Source: CAD feature listing. Evaluate the final solid. Frame: model axes, mm. A direction names the side the tool comes from. Round coordinates to 2 decimals unless told otherwise and drop trailing zeros. Order: outer loops, then holes, each group sorted by start corner. A loop starts at its lowest first (then second) coordinate and runs counter-clockwise, first axis right, second up. Notation, with made-up numbers: (-30, -17) - (-23, -17) arc R23 ccw to (-23, 0) - close; hole circle Ø2 at (84, 2). An arc over 180 degrees is marked (long way). Return JSON: item names as keys, results as strings. Group by question number.
1) Ray query, line 1 (Y direction, x = 32, z = 5); line 2 (X direction, y = 11, z = 5); line 3 (Y direction, x = 32, z = 8). Return the intervals inside material, ascending. Write a range as from..to.
2) Section C-C, the plane y = 10. Return loops of the section in (x, z), plus the area to 3 significant figures.
3) Section A-A, the plane z = 5.5. Give the number of separate pieces and of enclosed holes in the cut face, plus the area to 3 significant figures.
4) Section B-B, the plane y = 4. Return loops of the section in (x, z).
5) Access query for faces 4 (the flat face through (-4, 13, 3)), 5 (the flat face through (34, 13, 3)), 6 (the cylindrical face through (32, -2, 3)), 7 (the flat face through (30, 12, 3)). Directions: +Z, -Z, +X, -X, +Y, -Y. A direction counts if a zero-diameter tool reaches every point of the face in a straight line with its end or side. Return the directions, or none.
6) Section D-D, the plane x = -2. Return loops of the section in (y, z).
7) Contact query for flat-ended pins moving along their axis: P1, Ø3.5, axis at y = 12.5, z = 5, coming from the +X side; P2, Ø3, axis at x = 8, y = 23.5, coming from the -Z side; P3, Ø1, axis at x = 7.5, z = 5.5, coming from the +Y side. Output: stop coordinate, or through.
8) Mould query, pull axis Y, two halves, no side actions, for faces 1 (the cylindrical face through (-4.65, -4.49, 9.03)), 2 (the cylindrical face through (-0.5, 0.07, 5.42)), 3 (the flat face through (15, 32.5, 9)). Classes: pulls with the +Y half, pulls with the -Y half, needs draft (parallel to the pull), parting line crosses it, or undercut.
```python
from build123d import *

# Parameters (mm, degrees)
BOSS_EXTRUDE1_DEPTH   = 7
BOSS_EXTRUDE1_2_DEPTH = 7
SKETCH2_W             = 45
SKETCH2_H             = 40
BOSS_EXTRUDE2_DEPTH   = 4
FILLET1_R             = 10
SKETCH3_R             = 1.5
CUT_EXTRUDE1_DEPTH    = 16


with BuildPart() as part:
    # Sketch1 → Boss-Extrude1 (new body)
    with BuildSketch(Plane.XY):
        with BuildLine():
            Line((0, 0), (0, 25))
            ThreePointArc((0, 25), (-2, 27), (-4, 25))
            Line((-4, 25), (-4, 0))
            ThreePointArc((-4, 0), (-2, -2), (0, 0))
        make_face()
    extrude(amount=BOSS_EXTRUDE1_DEPTH)



with BuildPart() as body_2:
    # Sketch1 → Boss-Extrude1 2 (new body)
    with BuildSketch(Plane.XY):
        with BuildLine():
            Line((30, 0), (30, 25))
            ThreePointArc((30, 25), (32, 27), (34, 25))
            Line((34, 25), (34, 0))
            ThreePointArc((34, 0), (32, -2), (30, 0))
        make_face()
    extrude(amount=BOSS_EXTRUDE1_2_DEPTH)


with BuildPart() as part_1:
    add(part.part)

    add(body_2.part)  # Boss-Extrude2 merges body 2
    # Sketch2 → Boss-Extrude2 (add)
    with BuildSketch(Plane.XY.offset(7)):
        with Locations((15, 12.5)):
            Rectangle(SKETCH2_W, SKETCH2_H)
    extrude(amount=BOSS_EXTRUDE2_DEPTH)

    # Fillet1
    fillet1_edges = [part_1.edges().sort_by_distance(p)[0] for p in [
        (37.5, -7.5, 9),
        (37.5, 32.5, 9),
        (-7.5, 32.5, 9),
        (-7.5, -7.5, 9),
    ]]
    fillet(fillet1_edges, radius=FILLET1_R)

    # Sketch3 → Cut-Extrude1 (cut)
    with BuildSketch(Plane(origin=(0, 0, 0), x_dir=(-1, 0, 0), z_dir=(0, 0, -1))):
        with Locations((-32, 0)):
            Circle(SKETCH3_R)
        with Locations((-32, 4)):
            Circle(SKETCH3_R)
        with Locations((2, 0)):
            Circle(SKETCH3_R)
        with Locations((2, 4)):
            Circle(SKETCH3_R)
        with Locations((-32, 25)):
            Circle(SKETCH3_R)
        with Locations((-32, 21)):
            Circle(SKETCH3_R)
        with Locations((2, 25)):
            Circle(SKETCH3_R)
        with Locations((2, 21)):
            Circle(SKETCH3_R)
    extrude(amount=-CUT_EXTRUDE1_DEPTH, mode=Mode.SUBTRACT)


solid = part_1.part
```
Geometry check:
{
 "1": {"line 1": "-2..-1.5, 1.5..2.5, 5.5..19.5, 22.5..23.5, 26.5..27", "line 2": "-4..0, 30..34", "line 3": "-6.43..-1.5, 1.5..2.5, 5.5..19.5, 22.5..23.5, 26.5..31.43"},
 "2": {"outline": "(-7.5, 7) - (-4, 7) - (-4, 0) - (0, 0) - (0, 7) - (30, 7) - (30, 0) - (34, 0) - (34, 7) - (37.5, 7) - (37.5, 11) - (-7.5, 11) - close", "area": "236 mm2"},
 "3": {"separate pieces": "2", "enclosed holes": "8", "area": "169 mm2"},
 "4": {"outline": "(-7.5, 7) - (-4, 7) - (-4, 0) - (-3.5, 0) - (-3.5, 11) - (-7.5, 11) - close; (-0.5, 0) - (0, 0) - (0, 7) - (30, 7) - (30, 0) - (30.5, 0) - (30.5, 11) - (-0.5, 11) - close; (33.5, 0) - (34, 0) - (34, 7) - (37.5, 7) - (37.5, 11) - (33.5, 11) - close"},
 "5": {"face 4": "-Z, -X, +Y, -Y", "face 5": "-Z, +X, +Y, -Y", "face 6": "-Z, -Y", "face 7": "-Z, +Y, -Y"},
 "6": {"outline": "(-6.43, 7) - (-2, 7) - (-2, 0) - (-1.5, 0) - (-1.5, 11) - (-6.43, 11) - close; (1.5, 0) - (2.5, 0) - (2.5, 11) - (1.5, 11) - close; (5.5, 0) - (19.5, 0) - (19.5, 11) - (5.5, 11) - close; (22.5, 0) - (23.5, 0) - (23.5, 11) - (22.5, 11) - close; (26.5, 0) - (27, 0) - (27, 7) - (31.43, 7) - (31.43, 11) - (26.5, 11) - close"},
 "7": {"P1": "x = 34", "P2": "z = 7", "P3": "through"},
 "8": {"face 1": "pulls with the -Y half", "face 2": "undercut", "face 3": "pulls with the +Y half"}
}
